Geometry check sheet. Reference: the model listing, model coordinates, mm. A direction names the side the tool comes from. Round coordinates to 2 decimals unless told otherwise and drop trailing zeros. Order: outer loops, then holes, each group sorted by start corner. A loop starts at its lowest first (then second) coordinate and runs counter-clockwise, first axis right, second up. Notation, with made-up numbers: (-21, 82) - (-17, 82) arc R18 ccw to (-17, 108) - close; hole circle Ø10 at (37, 62). An arc over 180 degrees is marked (long way). Use a Markdown table: item, result. Add a question column.
(1) Gauge pin test, flat ends, axial feed: P1, Ø2, axis at x = -58.5, z = 8.5, coming from the -Y side; P2, Ø1, axis at x = -77.5, z = 4, coming from the -Y side; P3, Ø6, axis at x = -62, z = 3.5, coming from the +Y side; P4, Ø3.5, axis at x = -87.5, y = -12.5, coming from the -Z side. Record the tip position at first contact, or that the pin passes through.
(2) Mould release check, pull along Z, two halves, no side actions. Record for faces 1 (the face through (-42, 0, -13)), 2 (the face through (-42, -18.5, -3)), 3 (the face through (-53.7, -10.4, 3.5)): released by +Z, released by -Z, zero draft, split by the parting line, or undercut.
(3) Access from +Z, -Z, +X, -X, +Y, -Y to the whole of each face (thin tool, end or side, straight path). Record for faces 4 (the face through (-84.054, -1.277, 7.888)), 5 (the face through (-42, 0, -6.5)), 6 (the face through (-87.493, 0.33, 12.916)), 7 (the face through (-70, 17.5, 3)), 8 (the face through (-70, -17.5, 3)).
(4) Thickness scan on line 1 along Y through (x, z) = (-87.5, 4); line 2 along Y through (x, z) = (-52.5, 4.25); line 3 along Z through (x, y) = (-40.5, -12.5). Record the ranges inside material, lowest first. Write a range as [from, to].
(5) Section check C-C on y = -3.5. Record the boundary of the cut face in (x, z).
(6) Section check B-B on x = -52.5. Record the boundary of the cut face in (y, z), then the cut area to 3 significant figures.
(7) Section check A-A on y = 12.5. Record the boundary of the cut face in (x, z), then the cut area to 3 significant figures.
(8) Section check D-D on x = -80. Record the boundary of the cut face in (y, z), then the cut area to 3 significant figures.
```python
from build123d import *

# Parameters (mm, degrees)
SKETCH1_W           = 45
SKETCH1_H           = 35
SKETCH1_R           = 1.5
BOSS_EXTRUDE1_DEPTH = 7
SKETCH2_W           = 7
SKETCH2_H           = 50
BOSS_EXTRUDE2_DEPTH = 10
SKETCH3_W           = 10
SKETCH3_H           = 6.5
BOSS_EXTRUDE3_DEPTH = 6.5
SKETCH4_W           = 10
SKETCH4_H           = 50
BOSS_EXTRUDE4_DEPTH = 6.5
SKETCH5_R           = 7.5
BOSS_EXTRUDE5_DEPTH = 12
CUT_EXTRUDE1_DEPTH  = 16


with BuildPart() as part:
    # Sketch1 → Boss-Extrude1 (new body)
    with BuildSketch(Plane.XY):
        with Locations((-70, 0)):
            Rectangle(SKETCH1_W, SKETCH1_H)
        with Locations((-87.5, 12.5)):
            Circle(SKETCH1_R, mode=Mode.SUBTRACT)
        with Locations((-87.5, -12.5)):
            Circle(SKETCH1_R, mode=Mode.SUBTRACT)
        with Locations((-52.5, 9.5)):
            Circle(SKETCH1_R, mode=Mode.SUBTRACT)
        with Locations((-52.5, -9.5)):
            Circle(SKETCH1_R, mode=Mode.SUBTRACT)
    extrude(amount=BOSS_EXTRUDE1_DEPTH)

    # Sketch2 → Boss-Extrude2 (add)
    with BuildSketch(Plane(origin=(-47.5, 0, 0), x_dir=(0, 0, -1), z_dir=(1, 0, 0))):
        with Locations((-3.5, 0)):
            Rectangle(SKETCH2_W, SKETCH2_H)
    extrude(amount=BOSS_EXTRUDE2_DEPTH)

    # Sketch3 → Boss-Extrude3 (add)
    with BuildSketch(Plane(origin=(0, 0, 0), x_dir=(-1, 0, 0), z_dir=(0, 0, -1))):
        with Locations((42.5, 21.75)):
            Rectangle(SKETCH3_W, SKETCH3_H)
        with Locations((42.5, -21.75)):
            Rectangle(SKETCH3_W, SKETCH3_H)
    extrude(amount=BOSS_EXTRUDE3_DEPTH)

    # Sketch4 → Boss-Extrude4 (add)
    with BuildSketch(Plane(origin=(0, 0, -6.5), x_dir=(-1, 0, 0), z_dir=(0, 0, -1))):
        with Locations((42.5, 0)):
            Rectangle(SKETCH4_W, SKETCH4_H)
    extrude(amount=BOSS_EXTRUDE4_DEPTH)

    # Sketch5 → Boss-Extrude5 (add)
    with BuildSketch(Plane.XY.offset(7)):
        with Locations((-80, 0)):
            Circle(SKETCH5_R)
    extrude(amount=BOSS_EXTRUDE5_DEPTH)

    # Sketch1_3 → Cut-Extrude1 (cut)
    with BuildSketch(Plane.XY):
        with BuildLine():
            ThreePointArc((-75.75, 0), (-80, 4.25), (-84.25, 0))
            Line((-84.25, 0), (-75.75, 0))
        make_face()
        with BuildLine():
            Line((-75.75, 0), (-84.25, 0))
            ThreePointArc((-84.25, 0), (-80, -4.25), (-75.75, 0))
        make_face()
    extrude(amount=CUT_EXTRUDE1_DEPTH, mode=Mode.SUBTRACT)


solid = part.part
```
Check sheet entries:
| question | item | result |
|---|---|---|
| 1 | P1 | passes through |
| 1 | P2 | stops at y = -17.5 |
| 1 | P3 | stops at y = 17.5 |
| 1 | P4 | stops at z = 0 |
| 2 | face 1 | released by -Z |
| 2 | face 2 | undercut |
| 2 | face 3 | zero draft |
| 3 | face 4 | -Z |
| 3 | face 5 | +X, -X |
| 3 | face 6 | +Z |
| 3 | face 7 | +Z, -Z, -X, +Y |
| 3 | face 8 | +Z, -Z, -X, -Y |
| 4 | line 1 | y = [-17.5, -14], [-11, 11], [14, 17.5] |
| 4 | line 2 | y = [-17.5, -11], [-8, 8], [11, 17.5] |
| 4 | line 3 | z = [-13, -6.5], [0, 7] |
| 5 | outline | (-92.5, 0) - (-82.41, 0) - (-82.41, 16) - (-77.59, 16) - (-77.59, 0) - (-37.5, 0) - (-37.5, 7) - (-73.37, 7) - (-73.37, 19) - (-86.63, 19) - (-86.63, 7) - (-92.5, 7) - close; (-47.5, -13) - (-37.5, -13) - (-37.5, -6.5) - (-47.5, -6.5) - close |
| 6 | outline | (-17.5, 0) - (-11, 0) - (-11, 7) - (-17.5, 7) - close; (-8, 0) - (8, 0) - (8, 7) - (-8, 7) - close; (11, 0) - (17.5, 0) - (17.5, 7) - (11, 7) - close |
| 6 | area | 203 mm2 |
| 7 | outline | (-92.5, 0) - (-89, 0) - (-89, 7) - (-92.5, 7) - close; (-86, 0) - (-37.5, 0) - (-37.5, 7) - (-86, 7) - close; (-47.5, -13) - (-37.5, -13) - (-37.5, -6.5) - (-47.5, -6.5) - close |
| 7 | area | 429 mm2 |
| 8 | outline | (-17.5, 0) - (-4.25, 0) - (-4.25, 16) - (4.25, 16) - (4.25, 0) - (17.5, 0) - (17.5, 7) - (7.5, 7) - (7.5, 19) - (-7.5, 19) - (-7.5, 7) - (-17.5, 7) - close |
| 8 | area | 289 mm2 |
